Geometry check sheet. Reference: the model listing, model coordinates, mm. A direction names the side the tool comes from. Give positions to 0.01 mm unless a question says otherwise; leave off trailing zeros. Order: outer loops, then holes, each group sorted by start corner. A loop starts at its lowest first (then second) coordinate and runs counter-clockwise, first axis right, second up. Notation, with made-up numbers: M 60.5,18 L 106.5,18 A8 ccw 106.5,25 Z; hole C -21,12 d10. An arc over 180 degrees is marked long. Answer as a JSON object with one key per item and string values. Group by question number.
from build123d import *

# Parameters (mm, degrees)
SKETCH2_W           = 9.525
SKETCH2_H           = 9.525
BOSS_EXTRUDE1_DEPTH = 5.1816
CUT_EXTRUDE1_DEPTH  = 4.826


with BuildPart() as part:
    # Sketch1 → Revolve1 (revolve)
    with BuildSketch(Plane.XY, mode=Mode.PRIVATE) as revolve1_sk:
        Polygon((0, 3.175), (6.35, 3.175), (6.35, 1.5875), (12.7, 1.5875), (12.7, 0), (0, 0), align=None)
    revolve(revolve1_sk.sketch.rotate(Axis((0, 0, 0), (-1, 0, 0)), 90), axis=Axis((0, 0, 0), (-1, 0, 0)))

    # Sketch2 → Boss-Extrude1 (add)
    with BuildSketch(Plane(origin=(0, 0, 0), x_dir=(0, 0, -1), z_dir=(1, 0, 0))):
        Rectangle(SKETCH2_W, SKETCH2_H)
    extrude(amount=-BOSS_EXTRUDE1_DEPTH)

    # Sketch4 → Cut-Extrude1 (cut)
    with BuildSketch(Plane(origin=(12.7, 0, 0), x_dir=(0, 0, -1), z_dir=(1, 0, 0))):
        with BuildLine():
            Line((-1.371129549, -0.8001), (1.371129549, -0.8001))
            ThreePointArc((1.371129549, -0.8001), (0, -1.5875), (-1.371129549, -0.8001))
        make_face()
    extrude(amount=-CUT_EXTRUDE1_DEPTH, mode=Mode.SUBTRACT)


solid = part.part
1. Depth check by flat-ended pin: pin 1 (2 mm diameter, centred on x = 5, y = -3, fed in from +Z); pin 2 (2 mm diameter, centred on y = -2, z = -2.5, fed in from +X); pin 3 (1 mm diameter, centred on x = 6, z = -2.5, fed in from +Y). Enter the tip coordinate at first touch or a pass-through.
2. Cross-section at C-C (x = 11.5). Record the cut outline in (y, z) (1 decimal), and give its area (3 significant figures).
3. Thickness scan on line 1 along X through (y, z) = (-3.25, 0.75); line 2 along X through (y, z) = (-1, 1); line 3 along Y through (x, z) = (2.5, 2). Record the ranges inside material, lowest first. Write a range as [from, to].
4. Cross-section at D-D (y = -1). Record the cut outline in (x, z).
5. Access from +Z, -Z, +X, -X, +Y, -Y to the whole of each face (thin tool, end or side, straight path). Record for faces 1 (the cylindrical face through (3.22, 1.93, 2.52)), 2 (the flat face through (10, -0.8, 0)), 3 (the flat face through (-5.182, 0, 0)).
Report:
{
 "1": {"pin 1": "stops at z = 2.47", "pin 2": "stops at x = 6.35", "pin 3": "stops at y = 2.47"},
 "2": {"outline": "M -0.8,-1.4 A1.6 ccw long -0.8,1.4 Z", "area": "6.39 mm2"},
 "3": {"line 1": "x = [-5.18, 0]", "line 2": "x = [-5.18, 7.87]", "line 3": "y = [-2.47, 2.47]"},
 "4": {"outline": "M -5.18,-4.76 L 0,-4.76 L 0,-3.01 L 6.35,-3.01 L 6.35,-1.23 L 7.87,-1.23 L 7.87,1.23 L 6.35,1.23 L 6.35,3.01 L 0,3.01 L 0,4.76 L -5.18,4.76 Z"},
 "5": {"face 1": "+X", "face 2": "+Z, -Z, +X, -Y", "face 3": "+Z, -Z, -X, +Y, -Y"}
}
